```python
from build123d import *

# Parameters (mm, degrees)
F0_W     = 203.2
F0_H     = 203.2
F1_DEPTH = 4.7625
F3_DEPTH = 25.4
F5_D     = 9.525


with BuildPart() as f1:
    # F0 (on Front) → F1 (new body)
    with BuildSketch(Plane.XZ):
        with Locations((-69.8862, -6.438033)):
            Rectangle(F0_W, F0_H)
    extrude(amount=F1_DEPTH)

    # F2 (on face) → F3 (cut)
    with BuildSketch(Plane.XZ.offset(4.7625)):
        Polygon((31.7138, 95.161967), (-4.51766, 95.161967), (31.7138, 66.210844), align=None)
    extrude(amount=-F3_DEPTH, mode=Mode.SUBTRACT)

    # F5 (through all)
    with Locations(Plane.XZ.offset(4.7625)):
        with Locations((-164.311469, 88.123493), (-164.311469, -96.954145), (19.754818, -96.954145)):
            Hole(F5_D / 2)


solid = f1.part
```
Design review of the part built by this model. Coordinates are the model's own, in mm. Coordinates: 2 decimals unless noted, no trailing zeros. Write each loop counter-clockwise with the first axis right and the second up, starting at its lowest first coordinate (ties: lowest second). Pieces come first, ordered by that corner, then holes.
1) To check wall thickness, follow L1, parallel to X at y = -0.9, z = -95.5; L2, parallel to Z at x = 0.5, y = -0.65; L3, parallel to Z at x = -2, y = -0.95. State the ranges of each line that lie inside material, in increasing order.
2) Add section B-B (y = -1.7). Write out the cut boundary in (x, z) (1 decimal), plus the area to 3 significant figures.
3) Add section C-C (z = 71). Write out the cut boundary in (x, y).
4) Mouldability with a two-part tool opening along X and no side actions: class faces 1 (the flat face through (-171.486, -2, -8)), 2 (the cylindrical face through (20.37, -2.35, -92.23)), 3 (the flat face through (-71, -2, -108.038)) as +X half, -X half, draft (parallel to the pull), parting line (faces both ways), or undercut.
5) Add section A-A (x = 19.5). Write out the cut boundary in (y, z).
Check result:
1. L1: x = -171.49 to -168.85, -159.78 to 15.22, 24.29 to 31.71
1. L2: z = -108.04 to 91.15
1. L3: z = -108.04 to 93.15
2. outline: (-171.5, -108) - (31.7, -108) - (31.7, 66.2) - (-4.5, 95.2) - (-171.5, 95.2) - close; hole circle Ø9.5 at (-164.3, -97); hole circle Ø9.5 at (-164.3, 88.1); hole circle Ø9.5 at (19.8, -97)
2. area: 40,600 mm2
3. outline: (-171.49, -4.76) - (25.72, -4.76) - (25.72, 0) - (-171.49, 0) - close
4. face 1: -X half
4. face 2: undercut
4. face 3: draft
5. outline: (-4.76, -108.04) - (0, -108.04) - (0, -101.71) - (-4.76, -101.71) - close; (-4.76, -92.2) - (0, -92.2) - (0, 75.97) - (-4.76, 75.97) - close
